Here's how the part is built. I have some questions about the finished solid (model axes, mm). Face numbers are marked on the shaded views. A direction names the side the tool comes from. Round coordinates to 2 decimals unless told otherwise and drop trailing zeros. Loops run counter-clockwise (first coordinate to the right, second up) from the corner with the lowest first, then second, coordinate; pieces in that order, holes last. Notation, with made-up numbers: M 27.5,66 L 56.5,66 A28 ccw 56.5,105 Z; hole C -11.5,-38 d8. An arc over 180 degrees is marked long. Use a Markdown table: item, result.
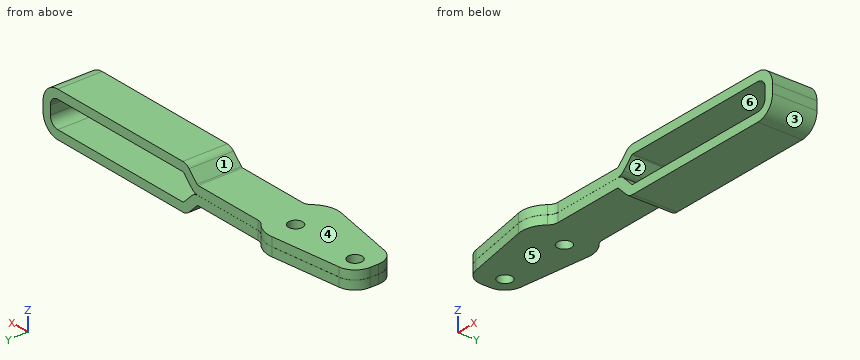
```python
from build123d import *

# Parameters (mm, degrees)
SKETCH1_W               = 133.35
SKETCH1_H               = 15.875
BASE_EXTRUDE_DEPTH      = 7.9375
CUT_EXTRUDE1_DEPTH      = 16.875
FILLET5_R               = 0.635
FILLET6_R               = 3.81
FILLET7_R               = 3.175
FILLET8_R               = 6.35
FILLET9_R               = 6.35
FILLET10_R              = 6.35
BOSS_EXTRUDE3_DEPTH     = 6.35
FILLET11_R              = 3.81
SKETCH7_R               = 2.54
CUT_EXTRUDE5_DEPTH      = 12.1125
SKETCH8_W               = 76.190653673
SKETCH8_H               = 0.0254
CUT_EXTRUDE6_DEPTH      = 4.175
CUT_EXTRUDE6_DEPTH_BACK = 21.447
FILLET12_R              = 3.81
FILLET13_R              = 3.81


with BuildPart() as part:
    # Sketch1 → Base-Extrude (new body, symmetric)
    with BuildSketch(Plane.XY):
        with Locations((66.675, 7.9375)):
            Rectangle(SKETCH1_W, SKETCH1_H)
    extrude(amount=BASE_EXTRUDE_DEPTH, both=True)

    # Sketch3 → Cut-Extrude1 (cut, through all)
    with BuildSketch(Plane(origin=(0, 15.875, 0), x_dir=(-1, 0, 0), z_dir=(0, 1, 0))):
        Polygon((-72.752628061, -4.7625), (-130.175, -4.7625), (-130.175, 4.7625), (-72.752628061, 4.7625), (-67.990128061, 0), align=None)
        Polygon((1.24743597, -3.175), (-66.675, -3.175), (-73.371059662, -9.871059662), (1.24743597, -9.871059662), align=None)
        Polygon((1.24743597, 3.175), (-66.675, 3.175), (-73.371059662, 9.871059662), (1.24743597, 9.871059662), align=None)
    extrude(amount=-CUT_EXTRUDE1_DEPTH, mode=Mode.SUBTRACT)

    # Fillet5
    fillet5_edges = [part.edges().sort_by_distance(p)[0] for p in [
        (72.752628061, 7.9375, -4.7625),
        (72.752628061, 7.9375, 4.7625),
        (66.675, 7.9375, 3.175),
        (66.675, 7.9375, -3.175),
    ]]
    fillet(fillet5_edges, radius=FILLET5_R)

    # Fillet6
    fillet6_edges = [part.edges().sort_by_distance(p)[0] for p in [
        (71.4375, 7.9375, -7.9375),
        (71.4375, 7.9375, 7.9375),
    ]]
    fillet(fillet6_edges, radius=FILLET6_R)

    # Fillet7
    fillet7_edges = [part.edges().sort_by_distance(p)[0] for p in [
        (130.175, 7.9375, -4.7625),
        (130.175, 7.9375, 4.7625),
    ]]
    fillet(fillet7_edges, radius=FILLET7_R)

    # Fillet8
    fillet8_edges = [part.edges().sort_by_distance(p)[0] for p in [
        (133.35, 7.9375, 7.9375),
        (133.35, 7.9375, -7.9375),
    ]]
    fillet(fillet8_edges, radius=FILLET8_R)

    # Fillet9
    fillet9_edges = [part.edges().sort_by_distance(p)[0] for p in [
        (0, 15.875, 0),
    ]]
    fillet(fillet9_edges, radius=FILLET9_R)

    # Fillet10
    fillet10_edges = [part.edges().sort_by_distance(p)[0] for p in [
        (0, 0, 0),
    ]]
    fillet(fillet10_edges, radius=FILLET10_R)

    # Sketch6 → Boss-Extrude3 (add)
    with BuildSketch(Plane.XY.offset(3.175)):
        with BuildLine():
            Line((5.564108911, 15.826180461), (30.825163366, 18.976770691))
            ThreePointArc((30.825163366, 18.976770691), (39.943880119, 14.786551928), (40.249024971, 4.755808431))
            ThreePointArc((40.249024971, 4.755808431), (36.72434383, -2.446073762), (28.949130797, -4.404784191))
            Line((28.949130797, -4.404784191), (5.165376283, 0.111477206))
            ThreePointArc((5.165376283, 0.111477206), (1.458943846, 2.300300048), (0, 6.35))
            Line((0, 6.35), (0, 9.525))
            ThreePointArc((0, 9.525), (1.590120358, 13.728099546), (5.564108911, 15.826180461))
        make_face()
    extrude(amount=-BOSS_EXTRUDE3_DEPTH)

    # Fillet11
    fillet11_edges = [part.edges().sort_by_distance(p)[0] for p in [
        (38.862, 0, 0),
        (39.103515829, 15.875, 0),
    ]]
    fillet(fillet11_edges, radius=FILLET11_R)

    # Sketch7 → Cut-Extrude5 (cut, through all)
    with BuildSketch(Plane.XY.offset(3.175)):
        with Locations((6.35, 9.525)):
            Circle(SKETCH7_R)
        with Locations((32.004, 9.525)):
            Circle(SKETCH7_R)
    extrude(amount=-CUT_EXTRUDE5_DEPTH, mode=Mode.SUBTRACT)

    # Sketch8 → Cut-Extrude6 (cut, two sides)
    with BuildSketch(Plane(origin=(0, 15.875, 0), x_dir=(-1, 0, 0), z_dir=(0, 1, 0))) as cut_extrude6_sk:
        with Locations((-34.920326837, 0)):
            Rectangle(SKETCH8_W, SKETCH8_H)
    extrude(amount=CUT_EXTRUDE6_DEPTH, mode=Mode.SUBTRACT)
    extrude(cut_extrude6_sk.sketch, amount=-CUT_EXTRUDE6_DEPTH_BACK, mode=Mode.SUBTRACT)

    # Fillet12
    fillet12_edges = [part.edges().sort_by_distance(p)[0] for p in [
        (68.002828061, 7.9375, 0.0127),
    ]]
    fillet(fillet12_edges, radius=FILLET12_R)

    # Fillet13
    fillet13_edges = [part.edges().sort_by_distance(p)[0] for p in [
        (68.002828061, 7.9375, -0.0127),
    ]]
    fillet(fillet13_edges, radius=FILLET13_R)


solid = part.part
```
Q1. Will these pins go through, and if not, where does the flat tip stop? P1, Ø5, axis at y = -1.5, z = -3, coming from the +X side; P2, Ø3, axis at x = 84.5, z = 3, coming from the -Y side; P3, Ø3, axis at x = 39.5, z = 1.5, coming from the +Y side; P4, Ø7, axis at x = 18.5, y = 1.5, coming from the -Z side (3 decimals).
Return value:
| item | result |
|---|---|
| P1 | stops at x = 133.35 |
| P2 | passes through |
| P3 | stops at y = 16.93 |
| P4 | stops at z = -3.175 |
Q2. We'd pull the mould along Z, two halves only. Please class the marked faces 1, 2 and 3: pulls with the +Z half, pulls with the -Z half, needs draft (parallel to the pull), parting line crosses it, or undercut.
Return value:
| item | result |
|---|---|
| face 1 | pulls with the +Z half |
| face 2 | undercut |
| face 3 | pulls with the -Z half |
Q3. For the marked faces 4, 5 and 6, which set-ups out of +Z, -Z, +X, -X, +Y, -Y let a thin tool reach every point of the face, with its end or its side?
Return value:
| item | result |
|---|---|
| face 4 | +Z, -X, +Y, -Y |
| face 5 | -Z, -X, +Y, -Y |
| face 6 | +Y, -Y |
Q4. Imagine slicing it at B-B, the plane x = 63.5. Please give me the cut outline in (y, z) (3 decimals).
Return value:
| item | result |
|---|---|
| outline | M 0,-3.175 L 15.875,-3.175 L 15.875,-0.013 L 0,-0.013 Z; M 0,0.013 L 15.875,0.013 L 15.875,3.175 L 0,3.175 Z |
Q5. I need wall thicknesses on line 1 (Z direction, x = 90, y = 1); line 2 (X direction, y = 8.75, z = -2.25); line 3 (Y direction, x = 97.5, z = 6) (3 decimals). Which ranges of each line are inside material? Lowest first, please. Write a range as from..to.
Return value:
| item | result |
|---|---|
| line 1 | z = -7.94..-4.76, 4.76..7.94 |
| line 2 | x = 0..3.93, 8.77..29.59, 34.42..70.24, 130.11..133.32 |
| line 3 | y = 0..15.875 |
Q6. Imagine slicing it at A-A, the plane x = 95. Please give me the cut outline in (y, z) (1 decimal).
Return value:
| item | result |
|---|---|
| outline | M 0,-7.9 L 15.9,-7.9 L 15.9,-4.8 L 0,-4.8 Z; M 0,4.8 L 15.9,4.8 L 15.9,7.9 L 0,7.9 Z |
